Check sheet for the drawn part. Datum: minimum x, y, z corner. Units: mm. Round coordinates to 2 decimals unless told otherwise and drop trailing zeros. Loops run counter-clockwise (first coordinate to the right, second up) from the corner with the lowest first, then second, coordinate; pieces in that order, holes last. Notation, with made-up numbers: (39.25, 26) -> (74.25, 26) arc R29 ccw to (74.25, 54) -> close; hole circle Ø3 at (-28.5, 59.25). An arc over 180 degrees is marked (long way). Use CSV: the item, a comma, the result in double quotes. Start each with the question number.
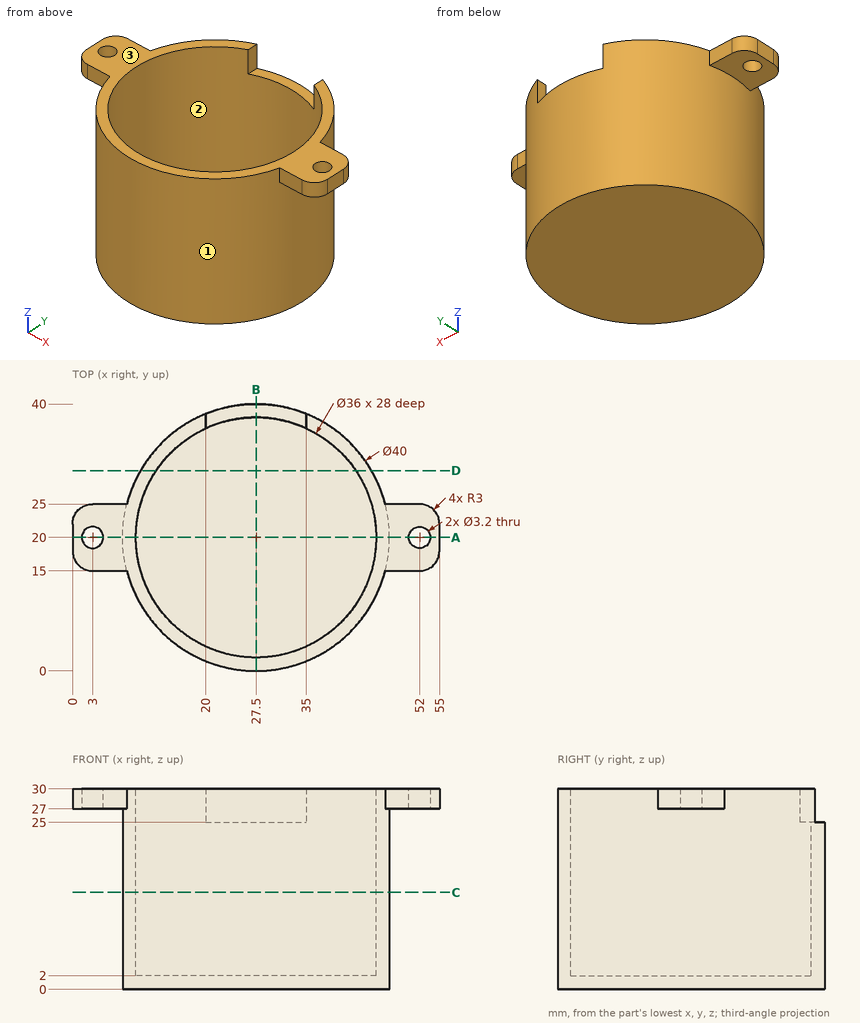
Q1. Cross-section at C-C (z = 14.5). Record the boundary of the cut face in (x, y).
Q2. Release check for a two-part mould opening along Y. For the marked faces 1, 2 and 3 record: +Y half, -Y half, draft (parallel to the pull), parting line (faces both ways), or undercut.
Q3. Thickness scan on L1, parallel to Y at x = 3, z = 28.4; L2, parallel to Y at x = 27.5, z = 15.5; L3, parallel to Z at x = 24, y = 29. Record the ranges inside material, lowest first. Write a range as from..to.
Q4. Depth check by flat-ended pin: pin 1 Ø5 at (x, y) = (44, 22.5) entering from +Z; pin 2 Ø4 at (x, y) = (28, 39) entering from +Z; pin 3 Ø8 at (y, z) = (33.5, 24) entering from -X; pin 4 Ø2.5 at (x, y) = (49.5, 17.5) entering from -Z. Enter the tip coordinate at first touch or a pass-through.
Q5. Cross-section at A-A (y = 20). Record the boundary of the cut face in (x, z).
Q6. Cross-section at D-D (y = 30). Record the boundary of the cut face in (x, z).
Q7. Cross-section at B-B (x = 27.5). Record the boundary of the cut face in (y, z), and give its area (3 significant figures).
Answer list:
1,outline,"circle Ø40 at (27.5, 20); hole circle Ø36 at (27.5, 20)"
2,face 1,"parting line"
2,face 2,"undercut"
2,face 3,"draft"
3,L1,"y = 15..18.4, 21.6..25"
3,L2,"y = 0..2, 38..40"
3,L3,"z = 0..2"
4,pin 1,"stops at z = 30"
4,pin 2,"stops at z = 25"
4,pin 3,"stops at x = 9.9"
4,pin 4,"stops at z = 27"
5,outline,"(0, 27) -> (1.4, 27) -> (1.4, 30) -> (0, 30) -> close; (4.6, 27) -> (7.5, 27) -> (7.5, 0) -> (47.5, 0) -> (47.5, 27) -> (50.4, 27) -> (50.4, 30) -> (45.5, 30) -> (45.5, 2) -> (9.5, 2) -> (9.5, 30) -> (4.6, 30) -> close; (53.6, 27) -> (55, 27) -> (55, 30) -> (53.6, 30) -> close"
6,outline,"(10.18, 0) -> (44.82, 0) -> (44.82, 30) -> (42.47, 30) -> (42.47, 2) -> (12.53, 2) -> (12.53, 30) -> (10.18, 30) -> close"
7,outline,"(0, 0) -> (40, 0) -> (40, 25) -> (38, 25) -> (38, 2) -> (2, 2) -> (2, 30) -> (0, 30) -> close"
7,area,"182 mm2"
